Input: part model. Units: mm. Frame: model coordinates. A direction names the side the tool comes from. Give positions to 0.01 mm unless a question says otherwise; leave off trailing zeros. One line per item, written item: value.
from build123d import *

# Parameters (mm, degrees)
SKETCH2_W           = 1057.275
SKETCH2_H           = 107.95
BOSS_EXTRUDE1_DEPTH = 22.225
SKETCH3_W           = 25.4
SKETCH3_H           = 82.55
BOSS_EXTRUDE2_DEPTH = 50.8
SKETCH4_R           = 6.35
CUT_EXTRUDE1_DEPTH  = 117.475
SKETCH5_W           = 3.175
SKETCH5_H           = 9.525
CUT_EXTRUDE2_DEPTH  = 1110.611399038
SKETCH6_R           = 12.7
CUT_EXTRUDE3_DEPTH  = 584.64108794


with BuildPart() as part:
    # Sketch2 → Boss-Extrude1 (new, symmetric)
    with BuildSketch(Plane.XY):
        Rectangle(SKETCH2_W, SKETCH2_H)
    extrude(amount=BOSS_EXTRUDE1_DEPTH, both=True)

    # Sketch3 → Boss-Extrude2 (add)
    with BuildSketch(Plane(origin=(528.6375, 0, 0), x_dir=(0, 0, -1), z_dir=(1, 0, 0))):
        Rectangle(SKETCH3_W, SKETCH3_H)
    boss_extrude2 = extrude(amount=BOSS_EXTRUDE2_DEPTH)

    # Sketch4 → Cut-Extrude1 (cut)
    with BuildSketch(Plane(origin=(579.4375, 0, 0), x_dir=(0, 0, -1), z_dir=(1, 0, 0))):
        Circle(SKETCH4_R)
    cut_extrude1 = extrude(amount=-CUT_EXTRUDE1_DEPTH, mode=Mode.SUBTRACT)

    # Mirror1: Boss-Extrude2, Cut-Extrude1 across plane
    add(boss_extrude2.mirror(Plane(origin=(0, 0, 0), x_dir=(0, 0, 1), z_dir=(1, 0, 0))))
    add(cut_extrude1.mirror(Plane(origin=(0, 0, 0), x_dir=(0, 0, 1), z_dir=(1, 0, 0))), mode=Mode.SUBTRACT)

    # Sketch5 → Cut-Extrude2 (cut, through all)
    with BuildSketch(Plane(origin=(528.6375, 0, 0), x_dir=(0, 0, -1), z_dir=(1, 0, 0))):
        with Locations((20.6375, 23.8125)):
            Rectangle(SKETCH5_W, SKETCH5_H)
    extrude(amount=-CUT_EXTRUDE2_DEPTH, mode=Mode.SUBTRACT)

    # Sketch6 → Cut-Extrude3 (cut, through all)
    with BuildSketch(Plane(origin=(0, 0, -22.225), x_dir=(-1, 0, 0), z_dir=(0, 0, -1))):
        with Locations((461.9625, 0)):
            Circle(SKETCH6_R)
        with Locations((-461.9625, 0)):
            Circle(SKETCH6_R)
    extrude(amount=-CUT_EXTRUDE3_DEPTH, mode=Mode.SUBTRACT)


solid = part.part
Item 1: Material intervals for L1, parallel to X at y = 1, z = 6.5; L2, parallel to Z at x = -516, y = 0 (3 decimals); L3, parallel to Z at x = -552.5, y = 0, sorted ascending.
Verdict:
L1: x = -579.44 to -474.62, -449.3 to 449.3, 474.62 to 579.44
L2: z = -22.225 to -6.35, 6.35 to 22.225
L3: z = -12.7 to -6.35, 6.35 to 12.7
Item 2: Draft query along X for faces 4 (the face through (579.438, 1, -8)), 5 (the face through (-449.275, 0.558, -0.311)), 6 (the face through (554, -1, -12.7)), 7 (the face through (449.849, 3.815, -0.311)). Return one class per face: pulls with the +X half, pulls with the -X half, needs draft (parallel to the pull), parting line crosses it, or undercut.
Verdict:
face 4: pulls with the +X half
face 5: undercut
face 6: needs draft
face 7: undercut
Item 3: Pin query (flat end, axial travel): P1, Ø7.5, axis at x = 565.5, z = 1, coming from the -Y side (3 decimals); P2, Ø15, axis at x = 559.5, y = -8.5, coming from the -Z side; P3, Ø5, axis at x = -223.5, y = 24, coming from the -Z side. Return the tip coordinate at first contact, or that it passes through.
Verdict:
P1: stops at y = -41.275
P2: stops at z = -12.7
P3: stops at z = -19.05
Item 4: Access query for faces 1 (the face through (554, -1, 12.7)), 2 (the face through (-554, -1, -12.7)), 3 (the face through (554, 41.275, 0)). Directions: +Z, -Z, +X, -X, +Y, -Y. A direction counts if a zero-diameter tool reaches every point of the face in a straight line with its end or side. Return the directions, or none.
Verdict:
face 1: +Z, +X, +Y, -Y
face 2: -Z, -X, +Y, -Y
face 3: +Z, -Z, +X, +Y
